Could you check a few things on this model? Use its own coordinates, in mm. A direction names the side the tool comes from. Give positions to 0.01 mm unless a question says otherwise; leave off trailing zeros. Loops run counter-clockwise (first coordinate to the right, second up) from the corner with the lowest first, then second, coordinate; pieces in that order, holes last. Notation, with made-up numbers: M 33,83.5 L 50,83.5 A17 cw 50,87.5 Z; hole C 39.25,-11 d1. An arc over 180 degrees is marked long. Answer in a Markdown table with one row per item. Add a question column.
1. I need wall thicknesses on line 1 along X through (y, z) = (-7.5, 6); line 2 along Y through (x, z) = (23.5, 44); line 3 along Y through (x, z) = (3, 40). Which ranges of each line are inside material? Lowest first, please. Write a range as from..to.
2. I'm going to push flat-ended pins straight in: pin 1 Ø4 at (x, z) = (0, 34.925) entering from +Y; pin 2 Ø8 at (x, y) = (-6.5, 11) entering from +Z. Where does each tip first touch, or does it pass through?
3. If we section it at A-A on z = 7.5: List the corners of the cut face in (x, y) for me, then the cut area to 3 significant figures.
4. Which directions (+Z, -Z, +X, -X, +Y, -Y) give clear straight access to the entire face, cutting with the end or side of a thin tool? Please do faces 1 (the flat face through (-1, 18.5, 25)), 2 (the cylindrical face through (0.035, 17.232, 42.862)), 3 (the flat face through (-3.167, 15, 38)), 4 (the flat face through (-1, -18.5, 25)), 5 (the cylindrical face through (-39.748, -14.787, 26.654)).
5. If we section it at C-C on y = -5.5: List the corners of the cut face in (x, z) for me (3 decimals).
6. If we section it at D-D on x = 11: List the corners of the cut face in (y, z) for me (3 decimals), then the cut area to 3 significant figures.
7. Thinking about a two-plate mould opening in Z: for faces 6 (the flat face through (-1, 13.5, 27)), 7 (the flat face through (1.588, 17, 39)), 8 (the flat face through (-2, 16, 41)), 9 (the flat face through (-1, -1, 3.175)), which applies, released by +Z, released by -Z, zero draft, split by the parting line, or undercut?
```python
from build123d import *

# Parameters (mm, degrees)
F0_W     = 87
F0_H     = 37
F1_DEPTH = 50.8
F2_W     = 81
F2_H     = 29
F3_DEPTH = 47.625
F4_R     = 2.5
F6_DEPTH = 2.5
F8_DEPTH = 25.4


with BuildPart() as f1:
    # F0 (on Top) → F1 (new body)
    with BuildSketch(Plane.XY):
        Rectangle(F0_W, F0_H)
    extrude(amount=F1_DEPTH)

    # F2 (on face) → F3 (cut)
    with BuildSketch(Plane.XY.offset(50.8)):
        with Locations((0, -1)):
            Rectangle(F2_W, F2_H)
    extrude(amount=-F3_DEPTH, mode=Mode.SUBTRACT)

    # F4
    f4_edges = [f1.edges().sort_by_distance(p)[0] for p in [
        (43.5, -18.5, 25.4),
        (-43.5, -18.5, 25.4),
        (-40.5, -15.5, 26.9875),
        (40.5, -15.5, 26.9875),
    ]]
    fillet(f4_edges, radius=F4_R)

    # F5 (on face) → F6 (cut)
    with BuildSketch(Plane.XZ.offset(-13.5)):
        with BuildLine():
            Line((3.166904, 35.151597), (3.166904, 41.048403))
            ThreePointArc((3.166904, 41.048403), (0.226597, 44.441904), (-3.166904, 41.501597))
            Line((-3.166904, 41.501597), (-3.166904, 41.048403))
            Line((-3.166904, 41.048403), (-3.166904, 35.151597))
            Line((-3.166904, 35.151597), (-3.166904, 34.698403))
            ThreePointArc((-3.166904, 34.698403), (0, 31.75), (3.166904, 34.698403))
            Line((3.166904, 34.698403), (3.166904, 35.151597))
        make_face()
        with BuildLine():
            Line((-3.166904, 41.048403), (-3.166904, 41.501597))
            ThreePointArc((-3.166904, 41.501597), (-3.175, 41.275), (-3.166904, 41.048403))
        make_face()
        with BuildLine():
            ThreePointArc((3.166904, 34.698403), (3.175, 34.925), (3.166904, 35.151597))
            Line((3.166904, 35.151597), (3.166904, 34.698403))
        make_face()
        with BuildLine():
            Line((-3.166904, 34.698403), (-3.166904, 35.151597))
            ThreePointArc((-3.166904, 35.151597), (-3.175, 34.925), (-3.166904, 34.698403))
        make_face()
    extrude(amount=-F6_DEPTH, mode=Mode.SUBTRACT)

    # F7 (on Front) → F8 (cut)
    with BuildSketch(Plane.XZ):
        with BuildLine():
            Line((-1.5875, 41.275), (-1.5875, 37.674631))
            ThreePointArc((-1.5875, 37.674631), (0, 31.75), (1.5875, 37.674631))
            Line((1.5875, 37.674631), (1.5875, 41.275))
            ThreePointArc((1.5875, 41.275), (0, 42.8625), (-1.5875, 41.275))
        make_face()
    extrude(amount=-F8_DEPTH, mode=Mode.SUBTRACT)


solid = f1.part
```
Results:
| question | item | result |
|---|---|---|
| 1 | line 1 | -43.5..-40.5, 40.5..43.5 |
| 1 | line 2 | -18.5..-15.5, 13.5..18.5 |
| 1 | line 3 | -18.5..-15.5, 16..18.5 |
| 2 | pin 1 | y = -15.5 |
| 2 | pin 2 | z = 50.8 |
| 3 | outline | M -43.5,-16 A2.5 ccw -41,-18.5 L 41,-18.5 A2.5 ccw 43.5,-16 L 43.5,18.5 L -43.5,18.5 Z; hole M -40.5,-13 A2.5 ccw -38,-15.5 L 38,-15.5 A2.5 ccw 40.5,-13 L 40.5,13.5 L -40.5,13.5 Z |
| 3 | area | 870 mm2 |
| 4 | face 1 | +Z, -Z, +X, -X, +Y |
| 4 | face 2 | +Y |
| 4 | face 3 | none |
| 4 | face 4 | +Z, -Z, +X, -X, -Y |
| 4 | face 5 | +Z |
| 5 | outline | M -43.5,0 L 43.5,0 L 43.5,50.8 L 40.5,50.8 L 40.5,3.175 L -40.5,3.175 L -40.5,50.8 L -43.5,50.8 Z |
| 6 | outline | M -18.5,0 L 18.5,0 L 18.5,50.8 L 13.5,50.8 L 13.5,3.175 L -15.5,3.175 L -15.5,50.8 L -18.5,50.8 Z |
| 6 | area | 498 mm2 |
| 7 | face 6 | zero draft |
| 7 | face 7 | undercut |
| 7 | face 8 | undercut |
| 7 | face 9 | released by +Z |
